Check sheet for the modelled part. Datum: model origin and axes. Units: mm. Face numbers are marked on the shaded views. A direction names the side the tool comes from. Give positions to 0.01 mm unless a question says otherwise; leave off trailing zeros. Order: outer loops, then holes, each group sorted by start corner. A loop starts at its lowest first (then second) coordinate and runs counter-clockwise, first axis right, second up.
Item 1: Release check for a two-part mould opening along X. For the marked faces 1, 2, 3 and 4 record: released by +X, released by -X, zero draft, split by the parting line, or undercut.
Item 2: Sectioned sample at A-A on x = 0. Record the boundary of the cut face in (y, z).
Item 3: Access from +Z, -Z, +X, -X, +Y, -Y to the whole of each face (thin tool, end or side, straight path). Record for the marked faces 5 and 6.
Item 4: Gauge pin test, flat ends, axial feed: P1, Ø1.5, axis at y = -5, z = 1.5, coming from the +X side; P2, Ø4, axis at x = -2, y = 0, coming from the +Z side; P3, Ø1, axis at x = 6, z = 13, coming from the +Y side. Record the tip position at first contact, or that the pin passes through.
Item 5: Material ranges on line 1 along Y through (x, z) = (0, 3.75); line 2 along Y through (x, z) = (0, 10.75); line 3 along Z through (x, y) = (8.75, -5.25), recorded low to high.
Item 6: Sectioned sample at C-C on z = 2. Record the boundary of the cut face in (x, y), and give its area (3 significant figures).
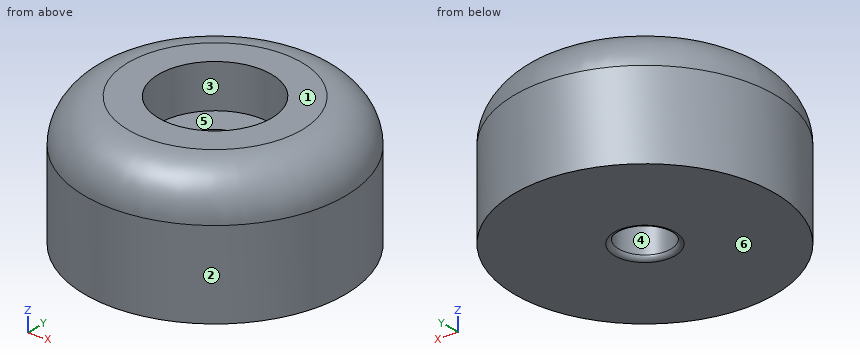
from build123d import *

# Parameters (mm, degrees)
IZIM1_R                     = 15
Y_KSEKLIK_EKSTR_ZYON1_DEPTH = 15
RADYUS1_R                   = 5
IZIM2_R                     = 3
KES_EKSTR_ZYON1_DEPTH       = 15
IZIM3_R                     = 6.5
KES_EKSTR_ZYON2_DEPTH       = 5
RADYUS2_R                   = 0.5


with BuildPart() as part:
    # Çizim1 → Yükseklik-Ekstrüzyon1 (new body)
    with BuildSketch(Plane.XY):
        Circle(IZIM1_R)
    extrude(amount=Y_KSEKLIK_EKSTR_ZYON1_DEPTH)

    # Radyus1
    radyus1_edges = [part.edges().sort_by_distance(p)[0] for p in [
        (-15, 0, 15),
    ]]
    fillet(radyus1_edges, radius=RADYUS1_R)

    # Çizim2 → Kes-Ekstrüzyon1 (cut)
    with BuildSketch(Plane(origin=(0, 0, 0), x_dir=(-1, 0, 0), z_dir=(0, 0, -1))):
        Circle(IZIM2_R)
    extrude(amount=-KES_EKSTR_ZYON1_DEPTH, mode=Mode.SUBTRACT)

    # Çizim3 → Kes-Ekstrüzyon2 (cut)
    with BuildSketch(Plane.XY.offset(15)):
        Circle(IZIM3_R)
    extrude(amount=-KES_EKSTR_ZYON2_DEPTH, mode=Mode.SUBTRACT)

    # Radyus2
    radyus2_edges = [part.edges().sort_by_distance(p)[0] for p in [
        (3, 0, 0),
    ]]
    fillet(radyus2_edges, radius=RADYUS2_R)


solid = part.part
Report:
1. face 1: zero draft
1. face 2: split by the parting line
1. face 3: undercut
1. face 4: undercut
2. outline: (-15, 0) - (-3.5, 0) arc R0.5 ccw to (-3, 0.5) - (-3, 10) - (-6.5, 10) - (-6.5, 15) - (-10, 15) arc R5 ccw to (-15, 10) - close; (3, 0.5) arc R0.5 ccw to (3.5, 0) - (15, 0) - (15, 10) arc R5 ccw to (10, 15) - (6.5, 15) - (6.5, 10) - (3, 10) - close
3. face 5: +Z
3. face 6: -Z, +X, -X, +Y, -Y
4. P1: stops at x = 14.39
4. P2: stops at z = 10
4. P3: stops at y = 13.08
5. line 1: y = -15 to -3, 3 to 15
5. line 2: y = -14.94 to -6.5, 6.5 to 14.94
5. line 3: z = 0 to 15
6. outline: circle Ø30 at (0, 0); hole circle Ø6 at (0, 0)
6. area: 679 mm2
